Here's how the part is built. I have some questions about the finished solid (model axes, mm). Face numbers are marked on the shaded views. Coordinates: 2 decimals unless noted, no trailing zeros. Write each loop counter-clockwise with the first axis right and the second up, starting at its lowest first coordinate (ties: lowest second). Pieces come first, ordered by that corner, then holes. Notation, with made-up numbers: (53.25, 26.25) -> (98.25, 26.25) arc R32 cw to (98.25, 61.25) -> close; hole circle Ø6 at (59, 14). An arc over 180 degrees is marked (long way). Put each result on its own line as item: value. Start each with the question number.
Item 1: I want a section at A-A, the plane z = 14.5. List the corners of the cut face in (x, y) for me, then the cut area to 3 significant figures.
Item 2: I need wall thicknesses on line 1 (Y direction, x = -208.5, z = 13.5); line 2 (X direction, y = -26.5, z = 22.25); line 3 (Y direction, x = -241, z = 21). Which ranges of each line are inside material? Lowest first, please. Write a range as [from, to].
Item 3: I want a section at C-C, the plane x = -44. List the corners of the cut face in (y, z) for me.
Item 4: I want a section at B-B, the plane y = -88. List the corners of the cut face in (x, z) for me.
Item 5: If we mould it in two halves opening along Y, with no side actions, what happens to the marked faces 1, 2 and 3? For each: released by +Y, released by -Y, zero draft, split by the parting line, or undercut.
from build123d import *

# Parameters (mm, degrees)
F0_W     = 364
F0_H     = 214
F1_DEPTH = 27
F3_DEPTH = 25
F4_W     = 360
F4_H     = 210
F5_DEPTH = 20
F6_DEPTH = 17


with BuildPart() as f1:
    # F0 (on Top) → F1 (new body)
    with BuildSketch(Plane.XY):
        with Locations((-182, -107)):
            Rectangle(F0_W, F0_H)
    extrude(amount=F1_DEPTH)

    # F2 (on face) → F3 (cut)
    with BuildSketch(Plane.XY.offset(27)):
        Polygon((-2, -2), (-246.590644, -2), (-362, -2), (-362, -107), (-362, -212), (-247.691646, -212), (-2, -212), (-2, -112.870261), align=None)
    extrude(amount=-F3_DEPTH, mode=Mode.SUBTRACT)

    # F4 (on face) → F5 (join)
    with BuildSketch(Plane.XY.offset(2)):
        with Locations((-182, -107)):
            Rectangle(F4_W, F4_H)
        Polygon((-357, -207), (-357, -107), (-357, -7), (-279.820502, -7), (-7, -7), (-7, -107), (-7, -207), (-279.820502, -207), align=None, mode=Mode.SUBTRACT)
    extrude(amount=F5_DEPTH)

    # F4 (on face) → F6 (cut)
    with BuildSketch(Plane.XY.offset(2)):
        with Locations((-182, -107)):
            Rectangle(F4_W, F4_H)
        Polygon((-357, -207), (-357, -107), (-357, -7), (-279.820502, -7), (-7, -7), (-7, -107), (-7, -207), (-279.820502, -207), align=None, mode=Mode.SUBTRACT)
    extrude(amount=F6_DEPTH, mode=Mode.SUBTRACT)


solid = f1.part
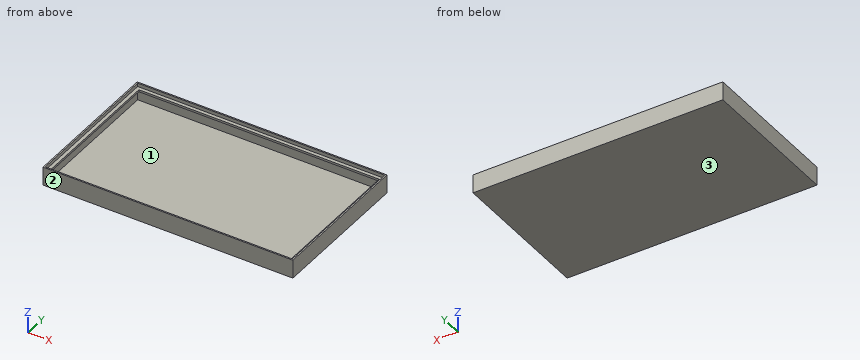
Calculated:
1. outline: (-364, -214) -> (0, -214) -> (0, 0) -> (-364, 0) -> close; hole (-362, -212) -> (-2, -212) -> (-2, -2) -> (-362, -2) -> close
1. area: 2,300 mm2
2. line 1: y = [-214, -212], [-2, 0]
2. line 2: x = [-364, -362], [-2, 0]
2. line 3: y = [-214, -207], [-7, 0]
3. outline: (-214, 0) -> (0, 0) -> (0, 27) -> (-2, 27) -> (-2, 22) -> (-7, 22) -> (-7, 19) -> (-2, 19) -> (-2, 2) -> (-212, 2) -> (-212, 19) -> (-207, 19) -> (-207, 22) -> (-212, 22) -> (-212, 27) -> (-214, 27) -> close
4. outline: (-364, 0) -> (0, 0) -> (0, 27) -> (-2, 27) -> (-2, 22) -> (-7, 22) -> (-7, 19) -> (-2, 19) -> (-2, 2) -> (-362, 2) -> (-362, 19) -> (-357, 19) -> (-357, 22) -> (-362, 22) -> (-362, 27) -> (-364, 27) -> close
5. face 1: undercut
5. face 2: released by -Y
5. face 3: zero draft
